Can you work these out from the drawing? Everything is in mm from the part's minimum corner. A direction names the side the tool comes from. Round coordinates to 2 decimals unless told otherwise and drop trailing zeros. Loops run counter-clockwise (first coordinate to the right, second up) from the corner with the lowest first, then second, coordinate; pieces in that order, holes last. Notation, with made-up numbers: (40.5, 21) -> (83.5, 21) arc R15 cw to (83.5, 39) -> close; hole circle Ø2 at (21, 77). An arc over 180 degrees is marked (long way). Answer as a JSON object with one key per item and string values.
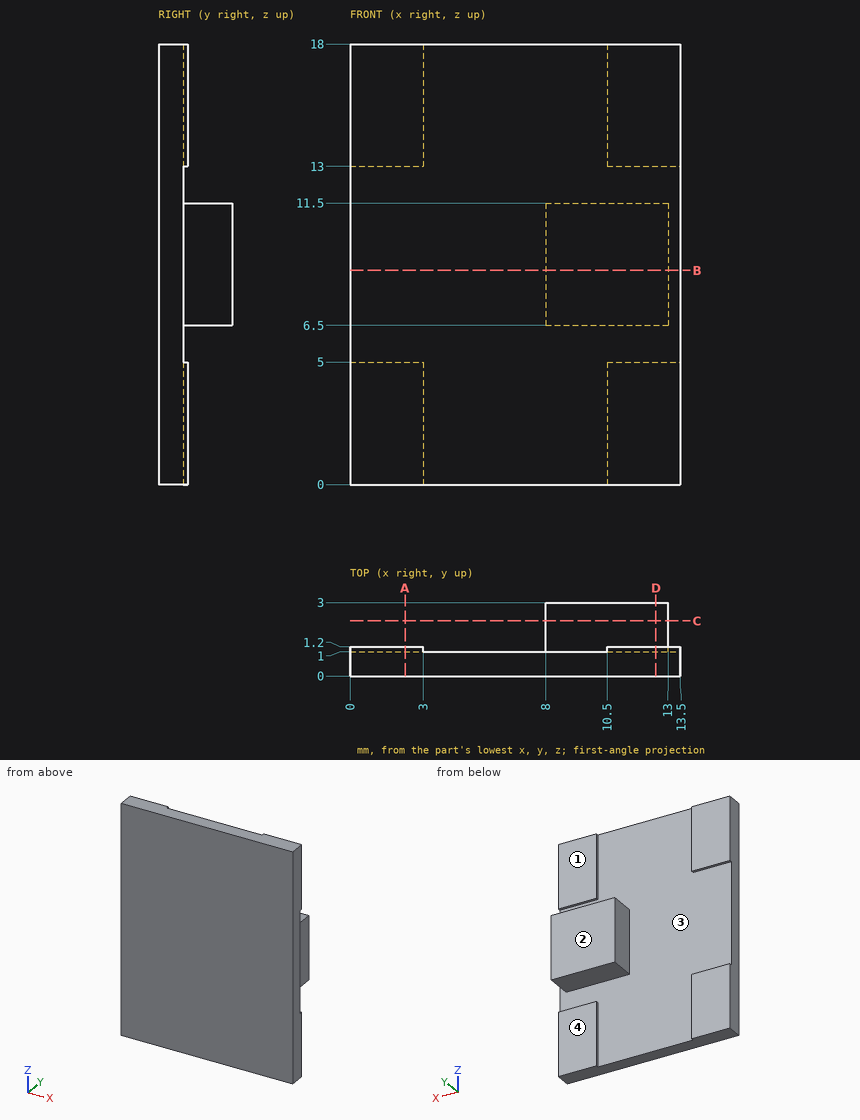
Q1. I want a section at A-A, the plane x = 2.25. Write out the boundary of the cut face in (y, z), then the cut area to 3 significant figures.
Determined:
{"outline": "(0, 0) -> (1.2, 0) -> (1.2, 5) -> (1, 5) -> (1, 13) -> (1.2, 13) -> (1.2, 18) -> (0, 18) -> close", "area": "20.0 mm²"}
Q2. On a 3-axis mill with a long thin cutter (end or side, diameter ignored), from which of +Z, -Z, +X, -X, +Y, -Y can I reach the whole of each face in a straight line? I mean the marked faces 1 and 2. Say none if no direction works.
Determined:
{"face 1": "+Z, +X, -X, +Y", "face 2": "+Z, -Z, +X, -X, +Y"}
Q3. I want a section at B-B, the plane z = 8.75. Write out the boundary of the cut face in (x, y), then the cut area to 3 significant figures.
Determined:
{"outline": "(0, 0) -> (13.5, 0) -> (13.5, 1) -> (13, 1) -> (13, 3) -> (8, 3) -> (8, 1) -> (0, 1) -> close", "area": "23.5 mm²"}
Q4. I'm going to push flat-ended pins straight in: pin 1 (3.5 mm diameter, centred on x = 1.5, z = 1.5, fed in from +Y); pin 2 (4 mm diameter, centred on x = 6, z = 6, fed in from +Y); pin 3 (0.6 mm diameter, centred on y = 2, z = 8.5, fed in from -X). Where does each tip first touch, or does it pass through?
Determined:
{"pin 1": "y = 1.2", "pin 2": "y = 1", "pin 3": "x = 8"}
Q5. If I drill on L1, parallel to Y at x = 5, z = 12.5; L2, parallel to X at y = 1.05, z = 2.25; L3, parallel to Z at x = 8.25, y = 1.7, over which ranges is the centre line in solid material (lowest first)? Write a range as [from, to].
Determined:
{"L1": "[0, 1]", "L2": "[0, 3], [10.5, 13.5]", "L3": "[6.5, 11.5]"}
Q6. I want a section at C-C, the plane y = 2.25. Write out the boundary of the cut face in (x, z), then the cut area to 3 significant figures.
Determined:
{"outline": "(8, 6.5) -> (13, 6.5) -> (13, 11.5) -> (8, 11.5) -> close", "area": "25.0 mm²"}
Q7. We'd pull the mould along X, two halves only. Please class the marked faces 3 and 4: pulls with the +X half, pulls with the -X half, needs draft (parallel to the pull), parting line crosses it, or undercut.
Determined:
{"face 3": "undercut", "face 4": "needs draft"}
Q8. I want a section at D-D, the plane x = 12.5. Write out the boundary of the cut face in (y, z).
Determined:
{"outline": "(0, 0) -> (1.2, 0) -> (1.2, 5) -> (1, 5) -> (1, 6.5) -> (3, 6.5) -> (3, 11.5) -> (1, 11.5) -> (1, 13) -> (1.2, 13) -> (1.2, 18) -> (0, 18) -> close"}
